The listing builds one solid part. Answer for the finished solid, in the listing's coordinates (mm). Coordinates: 2 decimals unless noted, no trailing zeros. Write each loop counter-clockwise with the first axis right and the second up, starting at its lowest first coordinate (ties: lowest second). Pieces come first, ordered by that corner, then holes.
from build123d import *

# Parameters (mm, degrees)
F0_R     = 11.15
F1_DEPTH = 7


with BuildPart() as f1:
    # F0 (on Front) → F1 (new body)
    with BuildSketch(Plane.XZ):
        with BuildLine():
            ThreePointArc((7.25, 19.245167), (12.557368, 24.552535), (14.5, 31.802535))
            ThreePointArc((14.5, 31.802535), (-7.25, 44.359903), (-7.25, 19.245167))
            ThreePointArc((-7.25, 19.245167), (0, 17.302535), (7.25, 19.245167))
        make_face()
        with Locations((0, 31.802535)):
            Circle(F0_R, mode=Mode.SUBTRACT)
        with BuildLine():
            ThreePointArc((7.25, 19.245167), (0, 17.302535), (-7.25, 19.245167))
            ThreePointArc((-7.25, 19.245167), (-8.842158, 12.634711), (-13.770902, 7.950634))
            ThreePointArc((-13.770902, 7.950634), (-18.699646, 3.266557), (-20.291803, -3.343899))
            ThreePointArc((-20.291803, -3.343899), (-14.984435, -8.651268), (-13.041803, -15.901268))
            ThreePointArc((-13.041803, -15.901268), (-6.520902, -13.974889), (0, -15.901268))
            ThreePointArc((0, -15.901268), (6.520902, -17.827646), (13.041803, -15.901268))
            ThreePointArc((13.041803, -15.901268), (14.984435, -8.651268), (20.291803, -3.343899))
            ThreePointArc((20.291803, -3.343899), (15.363059, 1.340178), (13.770902, 7.950634))
            ThreePointArc((13.770902, 7.950634), (12.178744, 14.56109), (7.25, 19.245167))
        make_face()
        Circle(F0_R, mode=Mode.SUBTRACT)
        with BuildLine():
            ThreePointArc((-13.041803, -15.901268), (-14.984435, -8.651268), (-20.291803, -3.343899))
            ThreePointArc((-20.291803, -3.343899), (-40.099172, -23.151268), (-13.041803, -15.901268))
        make_face()
        with Locations((-27.541803, -15.901268)):
            Circle(F0_R, mode=Mode.SUBTRACT)
        with BuildLine():
            ThreePointArc((42.041803, -15.901268), (34.791803, -3.343899), (20.291803, -3.343899))
            ThreePointArc((20.291803, -3.343899), (14.984435, -8.651268), (13.041803, -15.901268))
            ThreePointArc((13.041803, -15.901268), (27.541803, -30.401268), (42.041803, -15.901268))
        make_face()
        with Locations((27.541803, -15.901268)):
            Circle(F0_R, mode=Mode.SUBTRACT)
    extrude(amount=F1_DEPTH)


solid = f1.part
1. Section B-B on x = -2 is taken. Give the vertices of the cut face in (y, z), then the cut area to 3 significant figures.
Results found:
outline: (-7, -14.86) - (0, -14.86) - (0, -10.97) - (-7, -10.97) - close; (-7, 10.97) - (0, 10.97) - (0, 20.83) - (-7, 20.83) - close; (-7, 42.77) - (0, 42.77) - (0, 46.16) - (-7, 46.16) - close
area: 120 mm2
2. Section A-A on z = 41.5 is taken. Give the vertices of the cut face in (x, y), then the cut area to 3 significant figures.
Results found:
outline: (-10.78, -7) - (-5.5, -7) - (-5.5, 0) - (-10.78, 0) - close; (5.5, -7) - (10.78, -7) - (10.78, 0) - (5.5, 0) - close
area: 73.9 mm2
3. For a pull along Z with two mould halves and no side action, classify faces 1 (the flat face through (3, -7, 11)), 2 (the cylindrical face through (-38.68, -3.45, -15.41)), 3 (the cylindrical face through (6, -3.5, 41.2)) as pulls with the +Z half, pulls with the -Z half, needs draft (parallel to the pull), parting line crosses it, or undercut.
Results found:
face 1: needs draft
face 2: undercut
face 3: undercut
4. A flat-ended cylindrical pin translates along its axis: P1, Ø18, axis at x = -27.54, z = -15.9, coming from the -Y side. Find the tip coordinate at first contact, or state that the pin passes through.
Results found:
P1: passes through
5. Section D-D on z = -13 is taken. Give the vertices of the cut face in (x, y), then the cut area to 3 significant figures.
Results found:
outline: (-41.75, -7) - (-38.31, -7) - (-38.31, 0) - (-41.75, 0) - close; (-16.78, -7) - (16.78, -7) - (16.78, 0) - (-16.78, 0) - close; (38.31, -7) - (41.75, -7) - (41.75, 0) - (38.31, 0) - close
area: 283 mm2
6. Find the intervals of material crossed by L1, parallel to Z at x = -9, y = -0.75; L2, parallel to Z at x = -3.5, y = -4; L3, parallel to X at y = -1.25, z = -12.5, in increasing order.
Results found:
L1: z = -14.23 to -6.58, 6.58 to 12.37, 20.43 to 25.22, 38.38 to 43.17
L2: z = -14.36 to -10.59, 10.59 to 21.22, 42.39 to 45.87
L3: x = -41.64 to -38.16, -16.92 to 16.92, 38.16 to 41.64
7. Section C-C on x = 24 is taken. Give the vertices of the cut face in (y, z).
Results found:
outline: (-7, -29.96) - (0, -29.96) - (0, -26.47) - (-7, -26.47) - close; (-7, -5.33) - (0, -5.33) - (0, -1.84) - (-7, -1.84) - close
